Here's how the part is built. I have some questions about the finished solid (model axes, mm). A direction names the side the tool comes from. Round coordinates to 2 decimals unless told otherwise and drop trailing zeros. Order: outer loops, then holes, each group sorted by start corner. A loop starts at its lowest first (then second) coordinate and runs counter-clockwise, first axis right, second up. Notation, with made-up numbers: (6.5, 76) -> (20.5, 76) arc R9 cw to (20.5, 82) -> close; hole circle Ø2 at (-16, -11). An arc over 180 degrees is marked (long way). One line per item, written item: value.
```python
from build123d import *

# Parameters (mm, degrees)
F2_DEPTH = 16
F3_DEPTH = 12.6
F4_SIZE  = 2
F5_SIZE  = 0.6
F6_R     = 1.5
F7_DEPTH = 1
F7_TAPER = 45


with BuildPart() as f2:
    # F1 (on Top) → F2 (new body)
    with BuildSketch(Plane.XY):
        Polygon((-8, -5), (-2, -5), (-2, -3.5), (-4, -3.5), (-4, 3.5), (4, 3.5), (4, -3.5), (2, -3.5), (2, -5), (8, -5), (8, 5), (-8, 5), align=None)
        Polygon((-2, -3.5), (-2, -5), (2, -5), (2, -3.5), (4, -3.5), (4, 3.5), (-4, 3.5), (-4, -3.5), align=None)
    extrude(amount=F2_DEPTH)

    # F1 (on Top) → F3 (cut)
    with BuildSketch(Plane.XY):
        Polygon((-2, -3.5), (-2, -5), (2, -5), (2, -3.5), (4, -3.5), (4, 3.5), (-4, 3.5), (-4, -3.5), align=None)
    extrude(amount=F3_DEPTH, mode=Mode.SUBTRACT)

    # F4
    f4_edges = [f2.edges().sort_by_distance(p)[0] for p in [
        (-8, 0, 0),
        (-8, 0, 16),
        (8, 0, 16),
        (8, 0, 0),
    ]]
    chamfer(f4_edges, length=F4_SIZE)

    # F5
    f5_edges = [f2.edges().sort_by_distance(p)[0] for p in [
        (8, 5, 8),
        (7, 5, 1),
        (7, 5, 15),
        (0, 5, 0),
        (0, 5, 16),
        (-7, 5, 1),
        (-7, 5, 15),
        (-8, 5, 8),
        (-4, -5, 0),
        (-7, -5, 1),
        (-2, -5, 6.3),
        (-8, -5, 8),
        (0, -5, 12.6),
        (-7, -5, 15),
        (2, -5, 6.3),
        (0, -5, 16),
        (4, -5, 0),
        (7, -5, 15),
        (7, -5, 1),
        (8, -5, 8),
    ]]
    chamfer(f5_edges, length=F5_SIZE)

    # F6 (on face) → F7 (join)
    with BuildSketch(Plane(origin=(0, 5, 0), x_dir=(-1, 0, 0), z_dir=(0, 1, 0))):
        with Locations((-2.906170112, 4)):
            Circle(F6_R)
        with Locations((2.906170112, 4)):
            Circle(F6_R)
        with Locations((4.7022820183, 9.527864045)):
            Circle(F6_R)
        with Locations((0, 12.94427191)):
            Circle(F6_R)
        with Locations((-4.7022820183, 9.527864045)):
            Circle(F6_R)
        with Locations((0, 8)):
            Circle(F6_R)
    extrude(amount=F7_DEPTH, taper=F7_TAPER)


solid = f2.part
```
Q1. For P1, Ø8, axis at x = -0.5, z = 5.5, coming from the +Y side; P2, Ø1, axis at x = 0.5, z = 11.5, coming from the -Y side; P3, Ø2, axis at x = 0.5, y = -2, coming from the -Z side; P4, Ø4.5, axis at x = 3, z = 7, coming from the +Y side, each with a flat end and sliding along its axis, tell me the tip position at first contact or that it passes through.
Answers:
P1: y = 6
P2: y = 3.5
P3: z = 12.6
P4: y = 5.75
Q2. I want a section at B-B on x = 0. Write out the boundary of the cut face in (y, z).
Answers:
outline: (-5, 13.2) -> (-4.4, 12.6) -> (3.5, 12.6) -> (3.5, 0) -> (4.4, 0) -> (5, 0.6) -> (5, 6.5) -> (6, 7.5) -> (6, 8.5) -> (5, 9.5) -> (5, 11.44) -> (6, 12.44) -> (6, 13.44) -> (5, 14.44) -> (5, 15.4) -> (4.4, 16) -> (-4.4, 16) -> (-5, 15.4) -> close
Q3. I need wall thicknesses on line 1 along X through (y, z) = (-2.5, 4.75); line 2 along Y through (x, z) = (3, 11.25); line 3 along Y through (x, z) = (-6.5, 3.5). Which ranges of each line are inside material? Lowest first, please.
Answers:
line 1: -8 to -4, 4 to 8
line 2: -5 to -3.5, 3.5 to 5
line 3: -5 to 5
Q4. I want a section at A-A on y = -0.75. Write out the boundary of the cut face in (x, z).
Answers:
outline: (-8, 2) -> (-6, 0) -> (-4, 0) -> (-4, 12.6) -> (4, 12.6) -> (4, 0) -> (6, 0) -> (8, 2) -> (8, 14) -> (6, 16) -> (-6, 16) -> (-8, 14) -> close
Q5. Which directions (+Z, -Z, +X, -X, +Y, -Y) give clear straight access to the entire face, cutting with the end or side of a thin tool? Please do faces 1 (the face through (0, 3.5, 6)), 2 (the face through (0, 5, 10)), 3 (the face through (2, -4, 6)).
Answers:
face 1: -Z
face 2: +Y
face 3: -Z, -Y
